For this review, take the finished solid that the model builds, in its own axes (mm). Face numbers are marked on the shaded views. A direction names the side the tool comes from. Coordinates: 2 decimals unless noted, no trailing zeros. Loops run counter-clockwise (first coordinate to the right, second up) from the corner with the lowest first, then second, coordinate; pieces in that order, holes last. Notation, with made-up numbers: M 65,-27.5 L 123,-27.5 A18 cw 123,6.5 Z; hole C 45,17 d11. An arc over 180 degrees is marked long. Answer as a JSON object with one key per item and string values. Group by question number.
Item 1: Add section A-A (z = 19.5). State the section outline as (x, y) points, then the cut area to 3 significant figures.
Item 2: Tool access review of the marked faces 1 and 2: name each direction out of +Z, -Z, +X, -X, +Y, -Y from which nothing blocks a thin tool from reaching the whole face with its end or side.
Item 3: Add section C-C (y = 47). State the section outline as (x, z) points.
Item 4: Insertion check: pin 1 (6 mm diameter, centred on y = 3.5, z = 5.5, fed in from -X); pin 2 (12 mm diameter, centred on x = 23.5, z = 21, fed in from -Y); pin 3 (2 mm diameter, centred on y = 17.5, z = 14, fed in from +X); pin 4 (4 mm diameter, centred on x = 29.5, y = 26, fed in from -Z). Each pin has a flat end and moves straight along its axis. Give the tip position at first contact, or say it passes through.
Item 5: Wall thickness on L1, parallel to X at y = 31, z = -5; L2, parallel to Y at x = 23.5, z = 1.5; L3, parallel to Y at x = 27.5, z = -15.5: over which ranges is each line inside the solid? List them lowest first. Write a range as from..to.
Item 6: Add section B-B (x = 9.5). State the section outline as (y, z) points, then the cut area to 3 significant figures.
Item 7: Mouldability with a two-part tool opening along X and no side actions: class the marked faces 3, 4 and 5 as +X half, -X half, draft (parallel to the pull), parting line (faces both ways), or undercut.
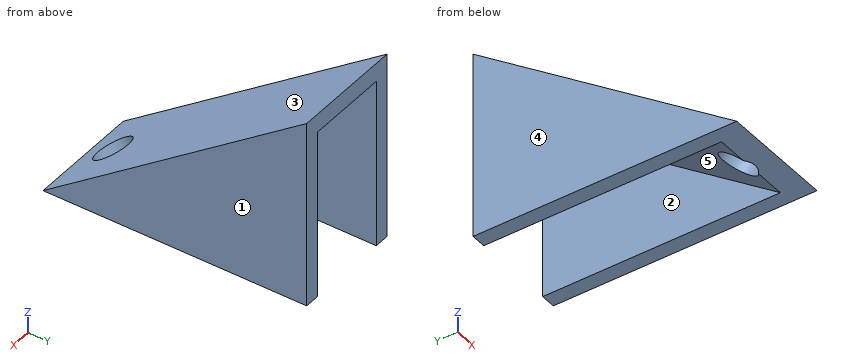
from build123d import *

# Parameters (mm, degrees)
F1_DEPTH       = 38.1
F2_T           = -5.08
F4_D           = 6.35
F4_CBORE_D     = 12.7
F4_CBORE_DEPTH = 5.08


with BuildPart() as f1:
    # F0 (on Right) → F1 (new body)
    with BuildSketch(Plane.YZ):
        Polygon((54.129655, 38.559098), (-34.77033, -24.890102), (54.129655, -24.940902), align=None)
    extrude(amount=F1_DEPTH)

    # F2
    f2_openings = [f1.faces().sort_by_distance(p)[0] for p in [
        (19.05, 9.679663, -24.915502),
        (19.05, 54.129655, 6.809098),
    ]]
    offset(amount=F2_T, openings=f2_openings)

    # F4 (through all)
    with Locations(Plane(origin=(0, 0.034999, -0.049037), x_dir=(1, 0, 0), z_dir=(0, -0.58093, 0.813953))):
        with Locations((19.05, -30.451737)):
            CounterBoreHole(F4_D / 2, F4_CBORE_D / 2, F4_CBORE_DEPTH)


solid = f1.part
From the geometry:
{
 "1": {"outline": "M 0,27.43 L 38.1,27.43 L 38.1,54.13 L 33.02,54.13 L 33.02,36.17 L 5.08,36.17 L 5.08,54.13 L 0,54.13 Z", "area": "516 mm²"},
 "2": {"face 1": "+Z, -Z, +X, +Y, -Y", "face 2": "-Z, +Y"},
 "3": {"outline": "M 0,-24.94 L 5.08,-24.94 L 5.08,27.23 L 33.02,27.23 L 33.02,-24.94 L 38.1,-24.94 L 38.1,33.47 L 0,33.47 Z"},
 "4": {"pin 1": "stops at x = 0", "pin 2": "stops at y = 21.12", "pin 3": "passes through", "pin 4": "stops at z = 10.81"},
 "5": {"L1": "x = 0..5.08, 33.02..38.1", "L2": "y = 2.21..10.95", "L3": "y = -21.61..-12.87"},
 "6": {"outline": "M -34.77,-24.89 L -26.03,-24.9 L 54.13,32.32 L 54.13,38.56 Z", "area": "528 mm²"},
 "7": {"face 3": "draft", "face 4": "-X half", "face 5": "undercut"}
}
